Model file for the job. Use its own axes, mm. Round coordinates to 2 decimals unless told otherwise and drop trailing zeros. Write each loop counter-clockwise with the first axis right and the second up, starting at its lowest first coordinate (ties: lowest second). Pieces come first, ordered by that corner, then holes. Notation, with made-up numbers: (58, 63) - (96, 63) arc R19 ccw to (96, 78) - close; hole circle Ø2 at (83.25, 16). An arc over 180 degrees is marked (long way). One line per item, written item: value.
from build123d import *

# Parameters (mm, degrees)
EXTRUDE_1_DEPTH = 5
SKETCH_2_R      = 1.25
EXTRUDE_4_DEPTH = 5


with BuildPart() as part:
    # 스케치1 → 보스-돌출1 (new body)
    with BuildSketch(Plane.XY):
        with BuildLine():
            Line((0, 10), (0, 37.192235936))
            ThreePointArc((0, 37.192235936), (3.845877906, 45.074290316), (12.42535625, 46.893660937))
            Line((12.42535625, 46.893660937), (152.42535625, 11.893660937))
            ThreePointArc((152.42535625, 11.893660937), (157.88205438, 8.34635803), (160, 2.192235936))
            Line((160, 2.192235936), (160, 0))
            Line((160, 0), (10, 0))
            ThreePointArc((10, 0), (2.928932188, 2.928932188), (0, 10))
        make_face()
    extrude(amount=EXTRUDE_1_DEPTH)

    # 스케치2 → 보스-돌출4 (add)
    with BuildSketch(Plane.XZ):
        with BuildLine():
            Line((150, 0), (139.801960973, 0))
            ThreePointArc((139.801960973, 0), (151.259085028, -7.924236418), (160.5, 2.5))
            ThreePointArc((160.5, 2.5), (151.259085028, 12.924236418), (139.801960973, 5))
            Line((139.801960973, 5), (150, 5))
            Line((150, 5), (160, 5))
            Line((160, 5), (160, 0))
            Line((160, 0), (150, 0))
        make_face()
        with Locations(Location((150, -4.37, 0), (0, 0, 270))):
            Circle(SKETCH_2_R, mode=Mode.SUBTRACT)
        with Locations(Location((150, 9.37, 0), (0, 0, 270))):
            Circle(SKETCH_2_R, mode=Mode.SUBTRACT)
    extrude(amount=-EXTRUDE_4_DEPTH)


solid = part.part
1. Band-saw the part on B-B on x = 46. Write the cut outline in (y, z), plus the area to 4 significant figures.
Report:
outline: (0, 0) - (38.5, 0) - (38.5, 5) - (0, 5) - close
area: 192.5 mm²
2. Mould opens along X. For faces 1 (the face through (160, 4, 3)), 2 (the face through (3.75, 45, 2.46)), 3 (the face through (150, 5, -2)) say: released by +X, released by -X, zero draft, split by the parting line, or undercut.
Report:
face 1: undercut
face 2: split by the parting line
face 3: zero draft
3. Wall check: probe 1 along Z at (x, y) = (150, 3.05); probe 2 along X at (y, z) = (3.35, 9.37); probe 3 along Z at (x, y) = (120, 11.5). Give the ranges that are in metal, low to high. Write a range as [from, to].
Report:
probe 1: [-8, -5.62], [-3.12, 8.12], [10.62, 13]
probe 2: [142.06, 148.75], [151.25, 157.94]
probe 3: [0, 5]
4. Band-saw the part on A-A on y = 30.5. Write the cut outline in (x, z), plus the area to 3 significant figures.
Report:
outline: (0, 0) - (78, 0) - (78, 5) - (0, 5) - close
area: 390 mm²
5. Drop flat-ended pins along their axis: pin 1 (12 mm diameter, centred on x = 86.5, y = 40.5, fed in from -Z); pin 2 (3 mm diameter, centred on x = 33.5, y = 5.5, fed in from +Z); pin 3 (6 mm diameter, centred on x = 73, y = 33, fed in from -Z); pin 4 (12 mm diameter, centred on x = 109.5, z = -4.5, fed in from -Y). Give the stop position or say it passes through.
Report:
pin 1: through
pin 2: z = 5
pin 3: z = 0
pin 4: y = 0
